Input: part model. Units: mm. Frame: model coordinates. A direction names the side the tool comes from. Coordinates: 2 decimals unless noted, no trailing zeros. Loops run counter-clockwise (first coordinate to the right, second up) from the corner with the lowest first, then second, coordinate; pieces in that order, holes last.
(1) Section A-A, the plane y = 0. Return loops of the section in (x, z) (3 decimals), then the cut area to 3 significant figures.
(2) Line query: L1, parallel to Z at x = -0.5, y = -16.5; L2, parallel to Z at x = -16.5, y = -6; L3, parallel to X at y = -5, z = 16. Output: solid intervals per line, ascending.
(3) Section C-C, the plane z = 8. Return loops of the section in (x, y).
(4) Contact query for flat-ended pins moving along their axis: P1, Ø1.5, axis at y = 11.5, z = 21.5, coming from the +X side; P2, Ø6, axis at x = 13, y = -13.5, coming from the +Z side; P3, Ø10, axis at x = -2.5, z = 28.5, coming from the -Y side; P4, Ø12, axis at y = 1, z = 9.5, coming from the -X side. Output: stop coordinate, or through.
(5) Mould query, pull axis X, two halves, no side actions, for faces 1 (the face through (4, -16, 25.093)), 2 (the face through (-1.65, 12.58, 16.74)), 3 (the face through (14.549, -4.582, 32.635)). Classes: released by +X, released by -X, zero draft, split by the parting line, or undercut.
(6) Set-up query: faces 4 (the face through (4, -16, 18.787)), 5 (the face through (-15.12, 11.59, 2.73)). Return all of +Z, -Z, +X, -X, +Y, -Y with unobstructed straight access to the full face (end or side cutting, diameter ignored); none if empty.
(7) Section D-D, the plane z = 18. Return loops of the section in (x, y).
```python
from build123d import *

# Parameters (mm, degrees)
F2_R     = 12.688559
F3_DEPTH = 33.02


with BuildPart() as f1:
    # F0 (on Front) → F1 (revolve)
    with BuildSketch(Plane.XZ):
        Polygon((0, 33.02), (0, 0), (19.05, 0), (19.05, 5.386552), (15.875, 11.824134), (19.05, 11.824134), (15.875, 18.787236), (19.05, 18.787236), (15.875, 25.09344), (19.05, 25.09344), (15.059195, 33.02), align=None)
    revolve(axis=Axis((0, 0, 16.51), (0, 0, -1)))

    # F2 (on face) → F3 (cut, through all)
    with BuildSketch(Plane.XY.offset(33.02)):
        Circle(F2_R)
    extrude(amount=-F3_DEPTH, mode=Mode.SUBTRACT)


solid = f1.part
```
Report:
1. outline: (-19.05, 0) - (-12.689, 0) - (-12.689, 33.02) - (-15.059, 33.02) - (-19.05, 25.093) - (-15.875, 25.093) - (-19.05, 18.787) - (-15.875, 18.787) - (-19.05, 11.824) - (-15.875, 11.824) - (-19.05, 5.387) - close; (12.689, 0) - (19.05, 0) - (19.05, 5.387) - (15.875, 11.824) - (19.05, 11.824) - (15.875, 18.787) - (19.05, 18.787) - (15.875, 25.093) - (19.05, 25.093) - (15.059, 33.02) - (12.689, 33.02) - close
1. area: 326 mm2
2. L1: z = 0 to 10.54, 11.82 to 17.4, 18.79 to 23.84, 25.09 to 30.14
2. L2: z = 0 to 8.41, 11.82 to 15.1, 18.79 to 21.75, 25.09 to 28.06
2. L3: x = -16.4 to -11.66, 11.66 to 16.4
3. outline: circle Ø35.52 at (0, 0); hole circle Ø25.38 at (0, 0)
4. P1: stops at x = 14.21
4. P2: stops at z = 31.66
4. P3: stops at y = -19.05
4. P4: stops at x = -19.05
5. face 1: zero draft
5. face 2: undercut
5. face 3: split by the parting line
6. face 4: none
6. face 5: +Z, -Z
7. outline: circle Ø32.47 at (0, 0); hole circle Ø25.38 at (0, 0)
